Can you work these out from the model? Positions are in its coordinate system, mm. Give positions to 0.01 mm unless a question says otherwise; leave off trailing zeros. Order: outer loops, then holes, each group sorted by start corner. A loop starts at its lowest first (then second) coordinate and runs counter-clockwise, first axis right, second up. Notation, with made-up numbers: (61.5, 1) - (109.5, 1) arc R21 cw to (109.5, 26) - close; hole circle Ø11 at (-5.75, 22). An arc over 180 degrees is marked (long way). One line per question, with ' | ' between items.
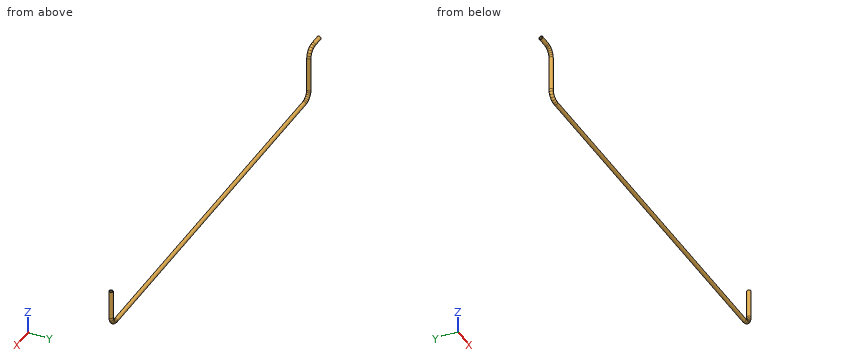
```python
from build123d import *

# Parameters (mm, degrees)
PROFILE_R   = 3.175
PROFILE_R_2 = 2.286


with BuildPart() as part:
    # Tube: sweep along a curve in space
    with BuildLine() as tube_path:
        Line((-3585.892778381, 0, 0), (-3567.692778381, 0, 0))
        Line((-3567.692778381, 0, 0), (-3563.810492704, 0, -0.511112606))
        Line((-3563.810492704, 0, -0.511112606), (-3560.192778381, 0, -2.009618943))
        Line((-3560.192778381, 0, -2.009618943), (-3557.086176663, 0, -4.393398282))
        Line((-3557.086176663, 0, -4.393398282), (-3554.702397324, 0, -7.5))
        Line((-3554.702397324, 0, -7.5), (-3553.203890986, 0, -11.117714323))
        Line((-3553.203890986, 0, -11.117714323), (-3552.692778381, 0, -15))
        Line((-3552.692778381, 0, -15), (-3552.692778381, 0, -73))
        Line((-3552.692778381, 0, -73), (-3552.181665775, 0, -76.882285677))
        Line((-3552.181665775, 0, -76.882285677), (-3550.683159438, 0, -80.5))
        Line((-3550.683159438, 0, -80.5), (-3548.299380099, 0, -83.606601718))
        Line((-3548.299380099, 0, -83.606601718), (-3545.192778381, 0, -85.990381057))
        Line((-3545.192778381, 0, -85.990381057), (-3541.575064057, 0, -87.488887394))
        Line((-3541.575064057, 0, -87.488887394), (-3537.692778381, 0, -88))
        Line((-3537.692778381, 0, -88), (-2926.592778381, 0, -88))
        Line((-2926.592778381, 0, -88), (-2922.710492704, 0, -87.488887394))
        Line((-2922.710492704, 0, -87.488887394), (-2919.092778381, 0, -85.990381057))
        Line((-2919.092778381, 0, -85.990381057), (-2915.986176663, 0, -83.606601718))
        Line((-2915.986176663, 0, -83.606601718), (-2913.602397324, 0, -80.5))
        Line((-2913.602397324, 0, -80.5), (-2912.103890986, 0, -76.882285677))
        Line((-2912.103890986, 0, -76.882285677), (-2911.592778381, 0, -73))
        Line((-2911.592778381, 0, -73), (-2911.592778381, 0, -25.3))
    # Profile → Tube (sweep)
    with BuildSketch(Plane(origin=(-3585.892778381, 0, 0), x_dir=(0, 0, -1), z_dir=(1, 0, 0))):
        Circle(PROFILE_R)
        Circle(PROFILE_R_2, mode=Mode.SUBTRACT)
    sweep(path=tube_path.line, transition=Transition.RIGHT)


solid = part.part
```
(1) Imagine slicing it at A-A (z = -33.5). List the corners of the cut face in (x, y) for me (3 decimals).
Answer below:
outline: circle Ø6.35 at (-3552.693, 0); circle Ø6.35 at (-2911.593, 0); hole circle Ø4.572 at (-3552.693, 0); hole circle Ø4.572 at (-2911.593, 0)
(2) If I drill on line 1 (X direction, y = 0.5, z = -56); line 2 (X direction, y = 0, z = -52.5); line 3 (Z direction, x = -3114.5, y = 0) (3 decimals), over which ranges is the centre line in solid material (lowest first)?
Answer below:
line 1: -3555.83 to -3554.92, -3550.46 to -3549.56, -2914.73 to -2913.82, -2909.36 to -2908.46 | line 2: -3555.87 to -3554.98, -3550.41 to -3549.52, -2914.77 to -2913.88, -2909.31 to -2908.42 | line 3: -91.175 to -90.286, -85.714 to -84.825
(3) Will these pins go through, and if not, where does the flat tip stop? pin 1 (1 mm diameter, centred on y = -1.5, z = -63, fed in from -X); pin 2 (2 mm diameter, centred on y = 0, z = -80.5, fed in from +X); pin 3 (3 mm diameter, centred on y = -1.5, z = -52, fed in from -X).
Answer below:
pin 1: x = -3555.71 | pin 2: x = -2909.75 | pin 3: x = -3555.87
(4) Imagine slicing it at B-B (x = -3294.5). List the corners of the cut face in (y, z) for me (3 decimals), and give its area (3 significant figures).
Answer below:
outline: circle Ø6.35 at (0, -88); hole circle Ø4.572 at (0, -88) | area: 15.3 mm^2
